```python
from build123d import *

# Parameters (mm, degrees)
SKETCH_R      = 1.75
SKETCH_R_2    = 2.75
PAD_DEPTH     = 3
SKETCH001_R   = 4
SKETCH001_R_2 = 1.75
PAD001_DEPTH  = 2
PAD002_DEPTH  = 1.6


with BuildPart() as part:
    # Sketch → Pad (new body)
    with BuildSketch(Plane.XY):
        Polygon((-70, 14.565403), (-70, -20), (70, -20), (70, 103.05), (61.165402, 103.05), align=None)
        with Locations((-63, 12.05)):
            Circle(SKETCH_R, mode=Mode.SUBTRACT)
        with Locations((-55, -10)):
            Circle(SKETCH_R_2, mode=Mode.SUBTRACT)
        with Locations((55, -10)):
            Circle(SKETCH_R_2, mode=Mode.SUBTRACT)
        with Locations((63, 12.05)):
            Circle(SKETCH_R, mode=Mode.SUBTRACT)
        with Locations((63, 97.05)):
            Circle(SKETCH_R, mode=Mode.SUBTRACT)
        with BuildLine():
            Line((-56, 6.05), (-7.5, 6.05))
            ThreePointArc((-7.45777, 4.050892), (-6.500223, 5.07112), (-7.5, 6.05))
            Line((-7.45777, 4.050892), (-55.95777, 2.000892))
            ThreePointArc((-57, 3), (-56.692015, 2.278117), (-55.95777, 2.000892))
            Line((-57, 3), (-57, 5.05))
            ThreePointArc((-56, 6.05), (-56.707107, 5.757107), (-57, 5.05))
        make_face(mode=Mode.SUBTRACT)
        with BuildLine():
            Line((56, 6.05), (7.5, 6.05))
            ThreePointArc((7.5, 6.05), (6.500223, 5.07112), (7.45777, 4.050892))
            Line((7.45777, 4.050892), (55.95777, 2.000892))
            ThreePointArc((55.95777, 2.000892), (56.692015, 2.278117), (57, 3))
            Line((57, 3), (57, 5.05))
            ThreePointArc((57, 5.05), (56.707107, 5.757107), (56, 6.05))
        make_face(mode=Mode.SUBTRACT)
        with BuildLine():
            Line((55.440753, 84.712883), (7.387406, 52.295942))
            ThreePointArc((7.387406, 52.295942), (6.946652, 51.466941), (7.387406, 50.63794))
            Line((7.387406, 50.63794), (55.440753, 18.220999))
            ThreePointArc((55.440753, 18.220999), (56.469443, 18.167037), (57, 19.05))
            Line((57, 19.05), (57, 83.883882))
            ThreePointArc((57, 83.883882), (56.469443, 84.766844), (55.440753, 84.712883))
        make_face(mode=Mode.SUBTRACT)
        with BuildLine():
            Line((-40.665942, 19.879001), (-5.129429, 43.852046))
            ThreePointArc((-4.010935, 43.852046), (-4.570182, 44.023045), (-5.129429, 43.852046))
            Line((-4.010935, 43.852046), (31.525578, 19.879001))
            ThreePointArc((30.966331, 18.05), (31.922627, 18.757597), (31.525578, 19.879001))
            Line((30.966331, 18.05), (-40.106695, 18.05))
            ThreePointArc((-40.665942, 19.879001), (-41.06299, 18.757597), (-40.106695, 18.05))
        make_face(mode=Mode.SUBTRACT)
    extrude(amount=PAD_DEPTH)

    # Sketch001 → Pad001 (join)
    with BuildSketch(Plane.XY.offset(3)):
        with Locations((-63, 12.05)):
            Circle(SKETCH001_R)
        with Locations((-63, 12.05)):
            Circle(SKETCH001_R_2, mode=Mode.SUBTRACT)
        with Locations((63, 12.05)):
            Circle(SKETCH001_R)
        with Locations((63, 12.05)):
            Circle(SKETCH001_R_2, mode=Mode.SUBTRACT)
        with Locations((63, 97.05)):
            Circle(SKETCH001_R)
        with Locations((63, 97.05)):
            Circle(SKETCH001_R_2, mode=Mode.SUBTRACT)
    extrude(amount=PAD001_DEPTH)

    # Sketch002 → Pad002 (join)
    with BuildSketch(Plane.XY.offset(3)):
        Polygon((64, 94.536369), (64, 15.524874), (59.525126, 11.05), (-60.864255, 11.05), (-61.788712, 14.07341), (60.35695, 96.473261), align=None)
        Polygon((60.348539, 94.055045), (-2.782063, 51.466941), (54.165402, 13.05), (59.127017, 13.05), (62, 15.922983), (62, 93.177017), align=None, mode=Mode.SUBTRACT)
        Polygon((-4.570182, 50.26067), (-59.230045, 13.386952), (-59.127017, 13.05), (50.589164, 13.05), align=None, mode=Mode.SUBTRACT)
    extrude(amount=PAD002_DEPTH)


solid = part.part
```
For this review, take the finished solid that the model builds, in its own axes (mm). A direction names the side the tool comes from. Give positions to 0.01 mm unless a question says otherwise; leave off trailing zeros. Write each loop counter-clockwise with the first axis right and the second up, starting at its lowest first coordinate (ties: lowest second). Pieces come first, ordered by that corner, then holes. Notation, with made-up numbers: M 54,54.25 L 76,54.25 A18 cw 76,83.25 Z; hole C 82,-1.75 d6. An arc over 180 degrees is marked long. One line per item, written item: value.
1) Take a section at B-B, the plane x = 26.5. Write out the cut boundary in (y, z), then the cut area to 3 significant figures.
Results are:
outline: M -20,0 L 3.25,0 L 3.25,3 L -20,3 Z; M 6.05,0 L 18.05,0 L 18.05,3 L 13.05,3 L 13.05,4.6 L 11.05,4.6 L 11.05,3 L 6.05,3 Z; M 23.27,0 L 37.74,0 L 37.74,3 L 31.71,3 L 31.71,4.6 L 29.3,4.6 L 29.3,3 L 23.27,3 Z; M 65.19,0 L 79.66,0 L 79.66,3 L 73.63,3 L 73.63,4.6 L 71.22,4.6 L 71.22,3 L 65.19,3 Z
area: 204 mm²
2) Take a section at D-D, the plane x = 44. Write out the cut boundary in (y, z), then the cut area to 3 significant figures.
Results are:
outline: M -20,0 L 2.51,0 L 2.51,3 L -20,3 Z; M 6.05,0 L 25.94,0 L 25.94,3 L 19.91,3 L 19.91,4.6 L 17.5,4.6 L 17.5,3 L 13.05,3 L 13.05,4.6 L 11.05,4.6 L 11.05,3 L 6.05,3 Z; M 76.99,0 L 91.47,0 L 91.47,3 L 85.44,3 L 85.44,4.6 L 83.03,4.6 L 83.03,3 L 76.99,3 Z
area: 182 mm²
3) For line 1 (Y direction, x = 55, z = 2.1); line 2 (Y direction, x = 41, z = 2.3); line 3 (Y direction, x = 44, z = 4.25), list the stretches that pass through material, from the lowest coordinate up. Write a range as from..to.
Results are:
line 1: y = -20..-12.75, -7.25..2.04, 6.05..18.52, 84.42..98.89
line 2: y = -20..2.63, 6.05..27.96, 74.97..89.45
line 3: y = 11.05..13.05, 17.5..19.91, 83.03..85.44
4) Take a section at A-A, the plane z = 1.5. Count the separate pieces of the cut face and the enclosed holes in it, then the cut area to 3 significant figures.
Results are:
separate pieces: 1
enclosed holes: 9
area: 8,290 mm²
5) For P1, Ø1.5, axis at y = 52, z = 1.5, coming from the -X side; P2, Ø0.8, axis at x = 56, z = 3.5, coming from the +Y side; P3, Ø1, axis at x = 63.5, y = 59, coming from the +Z side, all flat-tipped, find the tip position at first contact; note any pin that passes through.
Results are:
P1: stops at x = -15.62
P2: stops at y = 93.8
P3: stops at z = 4.6
6) The part is to be moulded in two halves that separate along Y. For faces 4 (the cylindrical face through (65.15, 100.423, 3.986)), 5 (the flat face through (31.37, 3.04, 1.48)), 6 (the flat face through (-1, -20, 1)), 7 (the flat face through (-70, -2, 1)), say which applies: +Y half, -Y half, draft (parallel to the pull), parting line (faces both ways), or undercut.
Results are:
face 4: undercut
face 5: undercut
face 6: -Y half
face 7: draft
7) Take a section at C-C, the plane y = -10. Write out the cut boundary in (x, z).
Results are:
outline: M -70,0 L -57.75,0 L -57.75,3 L -70,3 Z; M -52.25,0 L 52.25,0 L 52.25,3 L -52.25,3 Z; M 57.75,0 L 70,0 L 70,3 L 57.75,3 Z
8) For faces 1 (the cylindrical face through (-59.305, 10.518, 3.986)), 2 (the flat face through (15, 15, 0)), 3 (the flat face through (-31.37, 3.04, 1.48)), list the 3-axis set-ups (+Z, -Z, +X, -X, +Y, -Y) from which the entire face can be reached by the end or side of a thin tool; tool diameter is ignored.
Results are:
face 1: +Z
face 2: -Z, +X, -X, +Y, -Y
face 3: +Z, -Z
